Source: CAD feature listing. Evaluate the final solid. Frame: model axes, mm. Coordinates: 2 decimals unless noted, no trailing zeros. One line per question, with ' | ' between items. Start each with the question number.
(1) Contact query for flat-ended pins moving along their axis: P1, Ø2, axis at x = -36, z = 10, coming from the +Y side; P2, Ø1.5, axis at y = -7.5, z = 24, coming from the +X side; P3, Ø1.5, axis at y = -11, z = 45.5, coming from the -X side. Output: stop coordinate, or through.
(2) Draft query along X for faces 1 (the flat face through (-1, -9, 75)), 2 (the cylindrical face through (-0.867, -3.905, 36.975)). Return one class per face: +X half, -X half, draft (parallel to the pull), parting line (faces both ways), or undercut.
(3) Line query: line 1 along X through (y, z) = (-4.25, 9); line 2 along X through (y, z) = (-2.25, 36.5); line 3 along X through (y, z) = (5.9, 15). Output: solid intervals per line, ascending.
from build123d import *

# Parameters (mm, degrees)
SKETCH1_R           = 4
BOSS_EXTRUDE1_DEPTH = 75
SKETCH2_R           = 1
CUT_EXTRUDE1_DEPTH  = 75


with BuildPart() as part:
    # Sketch1 → Boss-Extrude1 (new body)
    with BuildSketch(Plane.XY):
        with BuildLine():
            ThreePointArc((7.5, 0), (0, 7.5), (-7.5, 0))
            add(Edge.make_bspline(
                [(-7.5, 0), (-13.133413819, -4.461912435), (-17.767441975, -11.345900192), (-26.448408985, -9.404150694)],
                knots=[0, 0, 0, 0, 1, 1, 1, 1], degree=3))
            add(Edge.make_bspline(
                [(-26.448408985, -9.404150694), (-34.892519394, -8.241593996), (-42.998591866, -5.63640498), (-50, 0)],
                knots=[0.508532521, 0.508532521, 0.508532521, 0.508532521, 1, 1, 1, 1], degree=3))
            add(Edge.make_bspline(
                [(-56.270853764, -7.789505316), (-58.317034017, -4.120672935), (-55.963516082, 2.956586768), (-50, 0)],
                knots=[0, 0, 0, 0, 1, 1, 1, 1], degree=3))
            add(Edge.make_bspline(
                [(0, -20.140225697), (-1.00593636, -20.15524797), (-3.047640759, -20.191257315), (-7.361898098, -20.266311816), (-13.006626751, -20.313476944), (-20.051108834, -20.120955208), (-27.291030951, -19.487291375), (-34.664372738, -18.197237521), (-42.077214845, -16.015044344), (-48.172992704, -13.24242478), (-52.871586187, -10.367033149), (-55.170435724, -8.6753845), (-56.270853764, -7.789505316)],
                knots=[0.002895243, 0.002895243, 0.002895243, 0.002895243, 0.0625, 0.125, 0.25, 0.375, 0.5, 0.625, 0.75, 0.875, 0.9375, 1, 1, 1, 1], degree=3))
            add(Edge.make_bspline(
                [(0, -20.140225697), (1.00593636, -20.15524797), (3.047640759, -20.191257315), (7.361898098, -20.266311816), (13.006626751, -20.313476944), (20.051108834, -20.120955208), (27.291030951, -19.487291375), (34.664372738, -18.197237521), (42.077214845, -16.015044344), (48.172992704, -13.24242478), (52.871586187, -10.367033149), (55.170435724, -8.6753845), (56.270853764, -7.789505316)],
                knots=[0.002895243, 0.002895243, 0.002895243, 0.002895243, 0.0625, 0.125, 0.25, 0.375, 0.5, 0.625, 0.75, 0.875, 0.9375, 1, 1, 1, 1], degree=3))
            add(Edge.make_bspline(
                [(56.270853764, -7.789505316), (58.317034017, -4.120672935), (55.963516082, 2.956586768), (50, 0)],
                knots=[0, 0, 0, 0, 1, 1, 1, 1], degree=3))
            add(Edge.make_bspline(
                [(26.448408985, -9.404150694), (34.892519394, -8.241593996), (42.998591866, -5.63640498), (50, 0)],
                knots=[0.508532521, 0.508532521, 0.508532521, 0.508532521, 1, 1, 1, 1], degree=3))
            add(Edge.make_bspline(
                [(26.448408985, -9.404150694), (17.767441975, -11.345900192), (13.133413819, -4.461912435), (7.5, 0)],
                knots=[0.885469804, 0.885469804, 0.885469804, 0.885469804, 1.885469804, 1.885469804, 1.885469804, 1.885469804], degree=3))
        make_face()
        Circle(SKETCH1_R, mode=Mode.SUBTRACT)
    extrude(amount=BOSS_EXTRUDE1_DEPTH)

    # Sketch2 → Cut-Extrude1 (cut)
    with BuildSketch(Plane(origin=(0, 0, 0), x_dir=(1, 0, 0), z_dir=(0, 1, 0))):
        with Locations(Location((0, -15, 0), (0, 0, 90))):
            Circle(SKETCH2_R)
    extrude(amount=CUT_EXTRUDE1_DEPTH, mode=Mode.SUBTRACT)


solid = part.part
Response values:
1) P1: stops at y = -7.01 | P2: stops at x = 56.71 | P3: stops at x = -52.94
2) face 1: draft | face 2: undercut
3) line 1: x = -56.98 to -43.51, -12.31 to 12.31, 43.51 to 56.98 | line 2: x = -56.54 to -46.91, -10.11 to -3.31, 3.31 to 10.11, 46.91 to 56.54 | line 3: x = -4.63 to -1, 1 to 4.63
